Autodesk Inventor part; units mm, degrees
ref_plane "YZ Plane" through (0, 0, 0) normal (1, 0, 0) x (0, 1, 0)
ref_plane "XZ Plane" through (0, 0, 0) normal (0, 1, 0) x (-1, 0, 0)
ref_plane "XY Plane" through (0, 0, 0) normal (0, 0, 1) x (1, 0, 0)
sketch "Sketch1" plane through (0, 0, 0) normal (0, 0, 1) x (1, 0, 0)
  line L0 (-107, -91) -> (107, -91)
  line L1 (107, -91) -> (107, 91)
  line L2 (107, 91) -> (-107, 91)
  line L3 (-107, 91) -> (-107, -91)
  line L4 (-107, -91) -> (107, 91) construction
  line L5 (107, -91) -> (-107, 91) construction
  point P0 (0, 0)
  dimension "d0" = 214
  dimension "d1" = 182
extrude "Extrusion1" add sketch "Sketch1" along normal blind 5
sketch "Sketch2" plane through (0, 0, 0) normal (0, 0, -1) x (-1, 0, 0)
  circle A0 centre (-49.8, 26.07) radius 20
  line L0 (-107, -91) -> (-107, 91)
  line L1 (107, -91) -> (-107, -91)
  point P0 (0, 0)
  dimension "d4" = 57.2
  dimension "d5" = 40
  dimension "d6" = 117.07
extrude "Extrusion2" cut sketch "Sketch2" against normal blind 5
properties part number "tapa_arriba"
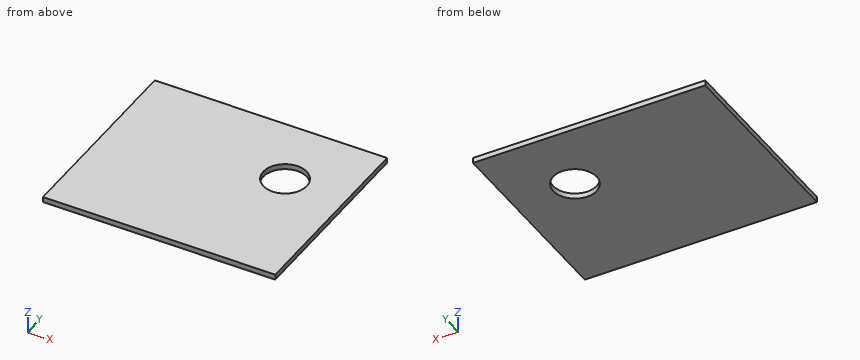
Model file for the job. Use its own axes, mm. Coordinates: 2 decimals unless noted, no trailing zeros. Write each loop counter-clockwise with the first axis right and the second up, starting at its lowest first coordinate (ties: lowest second). Pieces come first, ordered by that corner, then holes. Notation, with made-up numbers: (-25.5, -26.75) - (-3.5, -26.75) arc R25 ccw to (-3.5, -7.75) - close; hole circle Ø8 at (-23.5, 78). An arc over 180 degrees is marked (long way). Use a Markdown table: item, result. Add a question column.
Item 1: Drill centre lines: line 1 along Y through (x, z) = (49.8, 1.3); line 2 along Y through (x, z) = (56.5, 2.45). Where is each one in solid material? Low to high.
Item 2: Drop a flat-ended pin along its axis: pin 1 (3 mm diameter, centred on x = 66.5, y = 25, fed in from -Z). Give the stop position or say it passes through.
Item 3: Band-saw the part on B-B, the plane x = 49.8. Write the cut outline in (y, z).
Item 4: Band-saw the part on C-C, the plane z = 3.1. Write the cut outline in (x, y), and give its area (3 significant figures).
Item 5: Band-saw the part on A-A, the plane y = 26.07. Write the cut outline in (x, z).
A:
| question | item | result |
|---|---|---|
| 1 | line 1 | y = -91 to 6.07, 46.07 to 91 |
| 1 | line 2 | y = -91 to 7.23, 44.91 to 91 |
| 2 | pin 1 | passes through |
| 3 | outline | (-91, 0) - (6.07, 0) - (6.07, 5) - (-91, 5) - close; (46.07, 0) - (91, 0) - (91, 5) - (46.07, 5) - close |
| 4 | outline | (-107, -91) - (107, -91) - (107, 91) - (-107, 91) - close; hole circle Ø40 at (49.8, 26.07) |
| 4 | area | 37,700 mm² |
| 5 | outline | (-107, 0) - (29.8, 0) - (29.8, 5) - (-107, 5) - close; (69.8, 0) - (107, 0) - (107, 5) - (69.8, 5) - close |
